from build123d import *

# Parameters (mm, degrees)
SKETCH1_W                = 13
SKETCH1_H                = 38
SKETCH1_W_2              = 5
SKETCH1_H_2              = 30
BOSS_EXTRUDE1_DEPTH      = 4
CHAMFER1_SIZE            = 2
BOSS_EXTRUDE2_DEPTH      = 2
BOSS_EXTRUDE2_DEPTH_BACK = 2
SKETCH2_R                = 1.7
FILLET2_R                = 1


with BuildPart() as part:
    # Sketch1 → Boss-Extrude1 (new body)
    with BuildSketch(Plane.XY):
        Rectangle(SKETCH1_W, SKETCH1_H)
        Rectangle(SKETCH1_W_2, SKETCH1_H_2, mode=Mode.SUBTRACT)
    extrude(amount=BOSS_EXTRUDE1_DEPTH)

    # Chamfer1
    chamfer1_edges = [part.edges().sort_by_distance(p)[0] for p in [
        (-6.5, 19, 2),
        (6.5, 19, 2),
        (6.5, -19, 2),
        (-6.5, -19, 2),
    ]]
    chamfer(chamfer1_edges, length=CHAMFER1_SIZE)

    # Sketch2 → Boss-Extrude2 (add, two sides: drawn at the far end of the back side and taken through both)
    with BuildSketch(Plane.XY.offset(2).offset(-BOSS_EXTRUDE2_DEPTH_BACK)):
        Polygon((-6.5, 17), (-8.5, 15), (-24.5, 15), (-24.5, -15), (-8.5, -15), (-6.5, -17), align=None)
        with Locations((-16.5, 7.5)):
            Circle(SKETCH2_R, mode=Mode.SUBTRACT)
        with Locations((-16.5, -7.5)):
            Circle(SKETCH2_R, mode=Mode.SUBTRACT)
    extrude(amount=BOSS_EXTRUDE2_DEPTH + BOSS_EXTRUDE2_DEPTH_BACK)

    # Fillet2
    fillet2_edges = [part.edges().sort_by_distance(p)[0] for p in [
        (-2.5, -15, 2),
        (2.5, -15, 2),
        (2.5, 15, 2),
        (-2.5, 15, 2),
    ]]
    fillet(fillet2_edges, radius=FILLET2_R)


solid = part.part
Geometry check sheet. Reference: the model listing, model coordinates, mm. A direction names the side the tool comes from. Give positions to 0.01 mm unless a question says otherwise; leave off trailing zeros. Loops run counter-clockwise (first coordinate to the right, second up) from the corner with the lowest first, then second, coordinate; pieces in that order, holes last. Notation, with made-up numbers: M 5,65 L 23,65 A5 cw 23,73 Z; hole C 16.5,88.5 d10. An arc over 180 degrees is marked long. Answer as a JSON object with one key per item and string values. Group by question number.
Item 1: Mould release check, pull along X, two halves, no side actions. Record for faces 1 (the cylindrical face through (2.215, 14.699, 2.028)), 2 (the flat face through (-9, 0, 4)), 3 (the flat face through (-6.5, -17, 2)), 4 (the flat face through (5.5, -18, 2)): pulls with the +X half, pulls with the -X half, needs draft (parallel to the pull), parting line crosses it, or undercut.
Item 2: Material ranges on L1, parallel to Y at x = -16.5, z = 1.5; L2, parallel to X at y = -11, z = 2.3; L3, parallel to Y at x = -9.5, z = 1.4, recorded low to high.
Item 3: Sectioned sample at B-B on z = 3.2. Record the boundary of the cut face in (x, y).
Item 4: Sectioned sample at A-A on y = -7.5. Record the boundary of the cut face in (x, z), plus the area to 3 significant figures.
Item 5: Access from +Z, -Z, +X, -X, +Y, -Y to the whole of each face (thin tool, end or side, straight path). Record for faces 5 (the flat face through (-17, -15, 2)), 6 (the flat face through (-9, 0, 0)), 7 (the cylindrical face through (-2.199, -14.715, 2.028)).
Item 6: Sectioned sample at D-D on y = 10. Record the boundary of the cut face in (x, z), plus the area to 3 significant figures.
Item 7: Sectioned sample at C-C on x = -16.5. Record the boundary of the cut face in (y, z), plus the area to 3 significant figures.
Item 8: Gauge pin test, flat ends, axial feed: pin 1 (1 mm diameter, centred on x = -7.5, z = 2.5, fed in from -Y); pin 2 (1.2 mm diameter, centred on x = -12.5, z = 3, fed in from +Y). Record the tip position at first contact, or that the pin passes through.
Findings below:
{
 "1": {"face 1": "undercut", "face 2": "needs draft", "face 3": "pulls with the -X half", "face 4": "pulls with the +X half"},
 "2": {"L1": "-15 to -9.2, -5.8 to 5.8, 9.2 to 15", "L2": "-24.5 to -2.5, 2.5 to 6.5", "L3": "-15 to 15"},
 "3": {"outline": "M -24.5,-15 L -8.5,-15 L -4.5,-19 L 4.5,-19 L 6.5,-17 L 6.5,17 L 4.5,19 L -4.5,19 L -8.5,15 L -24.5,15 Z; hole C -16.5,-7.5 d3.4; hole C -16.5,7.5 d3.4; hole M -2.5,-14 A1 ccw -1.5,-15 L 1.5,-15 A1 ccw 2.5,-14 L 2.5,14 A1 ccw 1.5,15 L -1.5,15 A1 ccw -2.5,14 Z"},
 "4": {"outline": "M -24.5,0 L -18.2,0 L -18.2,4 L -24.5,4 Z; M -14.8,0 L -2.5,0 L -2.5,4 L -14.8,4 Z; M 2.5,0 L 6.5,0 L 6.5,4 L 2.5,4 Z", "area": "90.4 mm2"},
 "5": {"face 5": "+Z, -Z, -X, -Y", "face 6": "-Z, +X, -X, +Y, -Y", "face 7": "+Z, -Z"},
 "6": {"outline": "M -24.5,0 L -2.5,0 L -2.5,4 L -24.5,4 Z; M 2.5,0 L 6.5,0 L 6.5,4 L 2.5,4 Z", "area": "104 mm2"},
 "7": {"outline": "M -15,0 L -9.2,0 L -9.2,4 L -15,4 Z; M -5.8,0 L 5.8,0 L 5.8,4 L -5.8,4 Z; M 9.2,0 L 15,0 L 15,4 L 9.2,4 Z", "area": "92.8 mm2"},
 "8": {"pin 1": "y = -16.5", "pin 2": "y = 15"}
}
